from build123d import *

# Parameters (mm, degrees)
CYLINDER1036_R               = 1.5
CYLINDER1036_DEPTH           = 20
CYLINDER1034_R               = 1.5
CYLINDER1034_DEPTH           = 20
CYLINDER1031_R               = 1.5
CYLINDER1031_DEPTH           = 20
CYLINDER1035_R               = 1.5
CYLINDER1035_DEPTH           = 20
BOX431_W                     = 6
BOX431_H                     = 2
BOX431_DEPTH                 = 6
BOX432_W                     = 6
BOX432_H                     = 2
BOX432_DEPTH                 = 6
BOX430_W                     = 6
BOX430_H                     = 2
BOX430_DEPTH                 = 6
BOX429_W                     = 6
BOX429_H                     = 2
BOX429_DEPTH                 = 6
CYLINDER1038_R               = 4
CYLINDER1038_DEPTH           = 20
CYLINDER1038_PLACEMENT_ANGLE = 45
CYLINDER1037_R               = 4
CYLINDER1037_DEPTH           = 20
CYLINDER1037_PLACEMENT_ANGLE = 45
CYLINDER1032_R               = 10
CYLINDER1032_DEPTH           = 40
CYLINDER1039_R               = 10
CYLINDER1039_DEPTH           = 40
CYLINDER1033_R               = 52
CYLINDER1033_DEPTH           = 20
BOX433_W                     = 108
BOX433_H                     = 36
BOX433_DEPTH                 = 16
FILLET_R                     = 12


with BuildPart() as obj1:
    # Cylinder1036 → Cylinder1036 (new body)
    with BuildSketch(Plane(origin=(20, -40, -5), x_dir=(1, 0, 0), z_dir=(0, -1, 0))):
        Circle(CYLINDER1036_R)
    extrude(amount=CYLINDER1036_DEPTH)


with BuildPart() as obj2:
    # Cylinder1034 → Cylinder1034 (new body)
    with BuildSketch(Plane(origin=(51, -40, 7), x_dir=(1, 0, 0), z_dir=(0, -1, 0))):
        Circle(CYLINDER1034_R)
    extrude(amount=CYLINDER1034_DEPTH)


with BuildPart() as obj3:
    # Cylinder1031 → Cylinder1031 (new body)
    with BuildSketch(Plane(origin=(-51, -40, 7), x_dir=(1, 0, 0), z_dir=(0, -1, 0))):
        Circle(CYLINDER1031_R)
    extrude(amount=CYLINDER1031_DEPTH)


with BuildPart() as compound823:
    # Cylinder1035 → Cylinder1035 (new body)
    with BuildSketch(Plane(origin=(-20, -40, -5), x_dir=(1, 0, 0), z_dir=(0, -1, 0))):
        Circle(CYLINDER1035_R)
    extrude(amount=CYLINDER1035_DEPTH)

    # Compound823: union obj1, obj2, obj3
    add(obj1.part)
    add(obj2.part)
    add(obj3.part)


with BuildPart() as krychle431:
    # Box431 → Box431 (new body)
    with BuildSketch(Plane(origin=(17, -47, -8), x_dir=(1, 0, 0), z_dir=(0, 0, 1))):
        with Locations((3, 1)):
            Rectangle(BOX431_W, BOX431_H)
    extrude(amount=BOX431_DEPTH)


with BuildPart() as krychle432:
    # Box432 → Box432 (new body)
    with BuildSketch(Plane(origin=(48, -45, 4), x_dir=(1, 0, 0), z_dir=(0, 0, 1))):
        with Locations((3, 1)):
            Rectangle(BOX432_W, BOX432_H)
    extrude(amount=BOX432_DEPTH)


with BuildPart() as krychle430:
    # Box430 → Box430 (new body)
    with BuildSketch(Plane(origin=(-54, -45, 4), x_dir=(1, 0, 0), z_dir=(0, 0, 1))):
        with Locations((3, 1)):
            Rectangle(BOX430_W, BOX430_H)
    extrude(amount=BOX430_DEPTH)


with BuildPart() as compound824:
    # Box429 → Box429 (new body)
    with BuildSketch(Plane(origin=(-23, -47, -8), x_dir=(1, 0, 0), z_dir=(0, 0, 1))):
        with Locations((3, 1)):
            Rectangle(BOX429_W, BOX429_H)
    extrude(amount=BOX429_DEPTH)

    # Compound824: union Krychle431, Krychle432, Krychle430
    add(krychle431.part)
    add(krychle432.part)
    add(krychle430.part)


with BuildPart() as obj4:
    # Cylinder1038 → Cylinder1038 (new body)
    with BuildSketch(Plane.XY):
        Circle(CYLINDER1038_R)
    extrude(amount=CYLINDER1038_DEPTH)


with BuildPart() as obj4_1:
    # Cylinder1038 placement: moved
    add(obj4.part.moved(Location((39.6, -39.6, -10))).rotate(Axis((39.6, -39.6, -10), (0, 0, 1)), CYLINDER1038_PLACEMENT_ANGLE))


with BuildPart() as compound822:
    # Cylinder1037 → Cylinder1037 (new body)
    with BuildSketch(Plane.XY):
        Circle(CYLINDER1037_R)
    extrude(amount=CYLINDER1037_DEPTH)


with BuildPart() as compound822_1:
    # Cylinder1037 placement: moved
    add(compound822.part.moved(Location((-39.6, -39.6, -10))).rotate(Axis((-39.6, -39.6, -10), (0, 0, -1)), CYLINDER1037_PLACEMENT_ANGLE))

    # Compound822: union obj4
    add(obj4_1.part)


with BuildPart() as obj5:
    # Cylinder1032 → Cylinder1032 (new body)
    with BuildSketch(Plane(origin=(-59, -17, 0), x_dir=(1, 0, 0), z_dir=(0, 0, 1))):
        Circle(CYLINDER1032_R)
    extrude(amount=CYLINDER1032_DEPTH)


with BuildPart() as compound825:
    # Cylinder1039 → Cylinder1039 (new body)
    with BuildSketch(Plane(origin=(59, -17, 0), x_dir=(1, 0, 0), z_dir=(0, 0, 1))):
        Circle(CYLINDER1039_R)
    extrude(amount=CYLINDER1039_DEPTH)

    # Compound825: union obj5
    add(obj5.part)


with BuildPart() as obj6:
    # Cylinder1033 → Cylinder1033 (new body)
    with BuildSketch(Plane.XY.offset(20)):
        Circle(CYLINDER1033_R)
    extrude(amount=CYLINDER1033_DEPTH)


with BuildPart() as fillet_body:
    # Box433 → Box433 (new body)
    with BuildSketch(Plane(origin=(-54, -53, 20), x_dir=(1, 0, 0), z_dir=(0, 0, 1))):
        with Locations((54, 18)):
            Rectangle(BOX433_W, BOX433_H)
    extrude(amount=BOX433_DEPTH)

    # Cut432: cut obj6
    add(obj6.part, mode=Mode.SUBTRACT)


with BuildPart() as fillet_body_1:
    # Cut432 placement: moved
    add(fillet_body.part.moved(Location((0, 0, -20))))

    # Cut433: cut Compound825
    add(compound825.part, mode=Mode.SUBTRACT)

    # Cut431: cut Compound822
    add(compound822_1.part, mode=Mode.SUBTRACT)

    # Cut430: cut Compound824
    add(compound824.part, mode=Mode.SUBTRACT)

    # Cut429: cut Compound823
    add(compound823.part, mode=Mode.SUBTRACT)

    # Fillet
    fillet_edges = [fillet_body_1.edges().sort_by_distance(p)[0] for p in [
        (-54, -25.660254, 8),
        (54, -25.660254, 8),
    ]]
    fillet(fillet_edges, radius=FILLET_R)


solid = fillet_body_1.part
Read the model definition and answer for the solid it produces. Units are mm, in the model's axes. A direction names the side the tool comes from. Coordinates: 2 decimals unless noted, no trailing zeros. Order: outer loops, then holes, each group sorted by start corner. A loop starts at its lowest first (then second) coordinate and runs counter-clockwise, first axis right, second up. Notation, with made-up numbers: (-28, 86) - (0, 86) arc R14 cw to (0, 92) - close; hole circle Ø3 at (6.25, 13). An arc over 180 degrees is marked (long way). Use one line per item in the form item = value.
(1) Section C-C, the plane z = 13.25 is taken. Give the vertices of the cut face in (x, y).
Computed values:
outline = (-54, -53) - (54, -53) - (54, -30.96) arc R12 ccw to (51.27, -23.35) arc R10 cw to (49.01, -17.39) arc R52 cw to (-49.01, -17.39) arc R10 cw to (-51.27, -23.35) arc R12 ccw to (-54, -30.96) - close
(2) Straight lines are drawn through the part: L1, parallel to Z at x = -51, y = -49; L2, parallel to X at y = -39, z = 4.25; L3, parallel to X at y = -40.8, z = 7. For each, find the intervals that lie inside material, in ascending order.
Computed values:
L1 = 0 to 5.5, 8.5 to 16
L2 = -54 to -43.55, -35.65 to -34.39, 34.39 to 35.65, 43.55 to 54
L3 = -54 to -52.5, -49.5 to -43.42, -35.78 to -32.24, 32.24 to 35.78, 43.42 to 49.5, 52.5 to 54
(3) Section B-B, the plane x = -39 is taken. Give the vertices of the cut face in (y, z).
Computed values:
outline = (-53, 0) - (-43.55, 0) - (-43.55, 10) - (-35.65, 10) - (-35.65, 0) - (-34.39, 0) - (-34.39, 16) - (-53, 16) - close
(4) Which of the six approach directions +Z, -Z, +X, -X, +Y, -Y give full straight-line access (tool end or side, diameter ignored) to faces 4 (the face through (51, -40, 7)), 5 (the face through (-52.4, -45, 5.6)), 6 (the face through (51, -44, 10))?
Computed values:
face_4 = -Y
face_5 = -X
face_6 = +X
(5) Section A-A, the plane z = 7 is taken. Give the number of separate pieces and of enclosed holes in the cut face, then the cut area to 3 significant figures.
Computed values:
separate_pieces = 3
enclosed_holes = 2
area = 1,120 mm²
(6) Section D-D, the plane z = 2.75 is taken. Give the vertices of the cut face in (x, y), then the cut area to 3 significant figures.
Computed values:
outline = (-54, -53) - (54, -53) - (54, -30.96) arc R12 ccw to (51.27, -23.35) arc R10 cw to (49.01, -17.39) arc R52 cw to (-49.01, -17.39) arc R10 cw to (-51.27, -23.35) arc R12 ccw to (-54, -30.96) - close; hole circle Ø8 at (-39.6, -39.6); hole circle Ø8 at (39.6, -39.6)
area = 1,210 mm²
(7) Given pin 1 Ø3 at (x, z) = (17.5, 4) entering from +Y; pin 2 Ø1.8 at (x, z) = (51, 7) entering from +Y; pin 3 Ø4 at (x, y) = (38.5, -39.5) entering from -Z; pin 4 Ø10 at (x, y) = (-32, -27.5) entering from +Z, each flat-ended and moving along its own axis, determine where each tip first touches the part or whether it passes through.
Computed values:
pin_1 = -48.4
pin_2 = -21.56
pin_3 = 10
pin_4 = through
(8) For a pull along X with two mould halves and no side action, classify faces 1 (the face through (-52.2, -41.5, 6.1)), 2 (the face through (-54, -42, 8)), 3 (the face through (-13, -51, 16)) as pulls with the +X half, pulls with the -X half, needs draft (parallel to the pull), parting line crosses it, or undercut.
Computed values:
face_1 = undercut
face_2 = pulls with the -X half
face_3 = needs draft
